Part print with two shaded views. Sizes in mm from the minimum x, y, z corner. Give positions to 0.01 mm unless a question says otherwise; leave off trailing zeros. Order: outer loops, then holes, each group sorted by start corner. A loop starts at its lowest first (then second) coordinate and runs counter-clockwise, first axis right, second up.
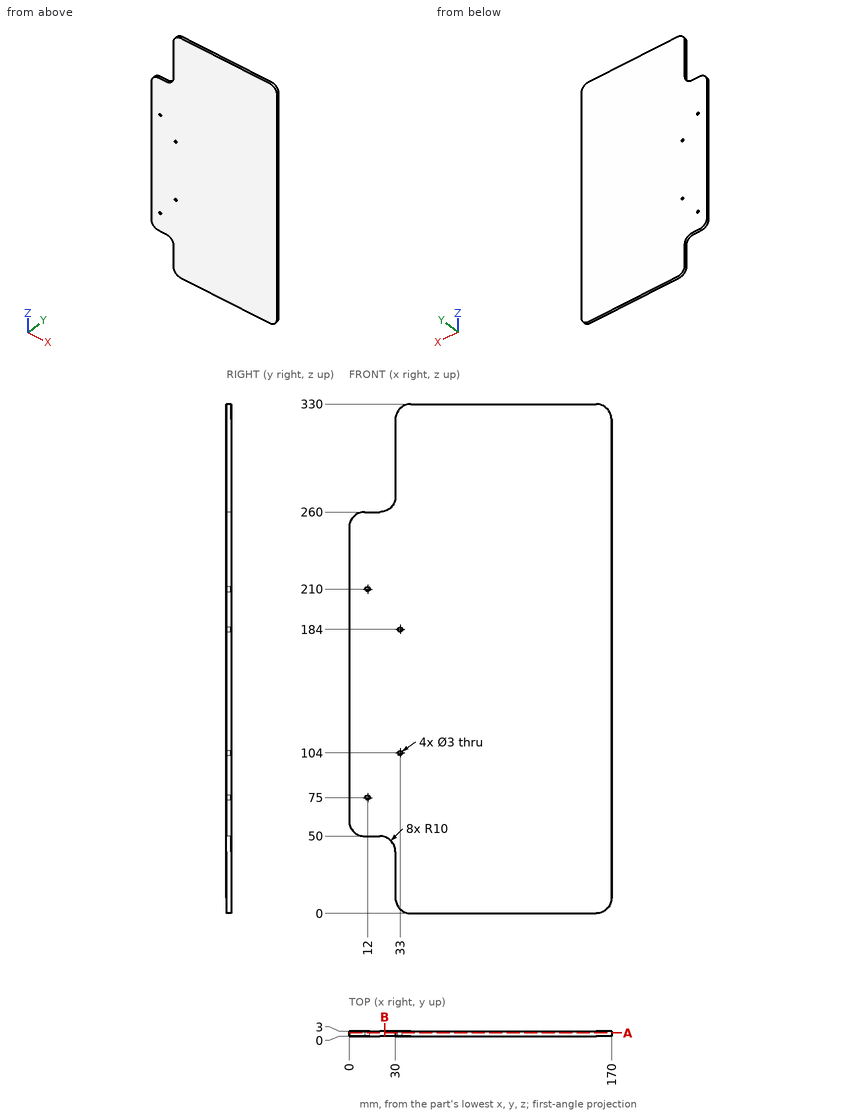
Item 1: Slice it at A-A (y = 2.1). Give the cut face in (x, z), and give its area (3 significant figures).
Item 2: Slice it at B-B (x = 23). Give the cut face in (y, z).
Item 3: Wall check: L1, parallel to X at y = 1.3, z = 75; L2, parallel to X at y = 2.25, z = 184; L3, parallel to Z at x = 9.5, y = 0.95. Give the ranges that are in metal, low to high.
Item 4: Drop flat-ended pins along their axis: pin 1 Ø1.8 at (x, z) = (12, 75) entering from +Y; pin 2 Ø0.9 at (y, z) = (1, 32) entering from -X; pin 3 Ø3.5 at (x, z) = (33, 184) entering from -Y. Give the stop position or say it passes through.
A:
1. outline: (0, 60) arc R10 ccw to (10, 50) - (20, 50) arc R10 cw to (30, 40) - (30, 10) arc R10 ccw to (40, 0) - (160, 0) arc R10 ccw to (170, 10) - (170, 320) arc R10 ccw to (160, 330) - (40, 330) arc R10 ccw to (30, 320) - (30, 270) arc R10 cw to (20, 260) - (10, 260) arc R10 ccw to (0, 250) - close; hole circle Ø3 at (12, 75); hole circle Ø3 at (12, 210); hole circle Ø3 at (33, 104); hole circle Ø3 at (33, 184)
1. area: 52,400 mm2
2. outline: (0, 49.54) - (3, 49.54) - (3, 260.46) - (0, 260.46) - close
3. L1: x = 0 to 10.5, 13.5 to 170
3. L2: x = 0 to 31.5, 34.5 to 170
3. L3: z = 50.01 to 259.99
4. pin 1: passes through
4. pin 2: stops at x = 30
4. pin 3: stops at y = 0
